Could you check a few things on this drawing? It's one solid part, dimensions in mm from its lowest x, y, z. Coordinates: 2 decimals unless noted, no trailing zeros. Loops run counter-clockwise (first coordinate to the right, second up) from the corner with the lowest first, then second, coordinate; pieces in that order, holes last. Notation, with made-up numbers: M 41,-36.75 L 47,-36.75 A23 cw 47,-3.75 Z; hole C 9.5,28 d11. An arc over 180 degrees is marked long. Use one line per item in the form item = value. Start each with the question number.
(1) Imagine slicing it at A-A, the plane z = 45.5. Please give me the cut outline in (x, y) (3 decimals), and give its area (3 significant figures).
(2) Please list where these lines run through material, in increasing order: L1, parallel to X at y = 7, z = 23; L2, parallel to Y at x = 24.5, z = 64.5 (3 decimals); L3, parallel to Z at x = 25.5, y = 6.75.
(3) Will these pins go through, and if not, where does the flat tip stop? P1, Ø2.5, axis at x = 25, y = 10.5, coming from the -Z side; P2, Ø2.5, axis at x = 25.5, z = 52, coming from the +Y side; P3, Ø8, axis at y = 8.5, z = 27, coming from the +X side.
(4) Imagine slicing it at B-B, the plane y = 11. Please give me the cut outline in (x, z).
(5) Imagine slicing it at C-C, the plane x = 25.5. Please give me the cut outline in (y, z) (3 decimals).
(6) Thinking about a two-plate mould opening in X: for the marked faces 1, 2 and 3, which applies, +X half, -X half, draft (parallel to the pull), parting line (faces both ways), or undercut?
(7) Imagine slicing it at D-D, the plane z = 24. Please give me the cut outline in (x, y), and give its area (3 significant figures).
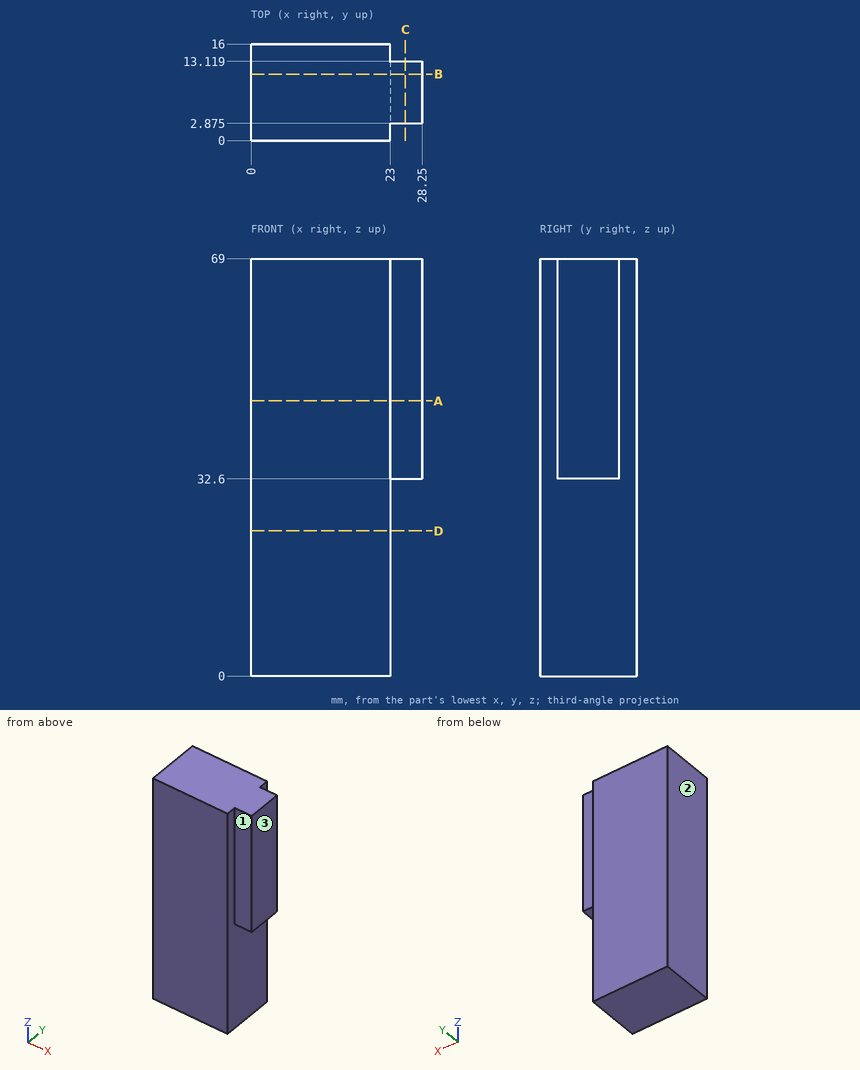
Answer:
q1.outline = M 0,0 L 23,0 L 23,2.875 L 28.25,2.875 L 28.25,13.119 L 23,13.119 L 23,16 L 0,16 Z
q1.area = 422 mm²
q2.L1 = 0 to 23
q2.L2 = 2.875 to 13.119
q2.L3 = 32.6 to 69
q3.P1 = 32.6
q3.P2 = 13.12
q3.P3 = 23
q4.outline = M 0,0 L 23,0 L 23,32.6 L 28.25,32.6 L 28.25,69 L 0,69 Z
q5.outline = M 2.875,32.6 L 13.119,32.6 L 13.119,69 L 2.875,69 Z
q6.face_1 = draft
q6.face_2 = -X half
q6.face_3 = +X half
q7.outline = M 0,0 L 23,0 L 23,16 L 0,16 Z
q7.area = 368 mm²
